Read the model definition and answer for the solid it produces. Units are mm, in the model's axes. Face numbers are marked on the shaded views. A direction names the side the tool comes from. Give positions to 0.01 mm unless a question says otherwise; leave off trailing zeros. Loops run counter-clockwise (first coordinate to the right, second up) from the corner with the lowest first, then second, coordinate; pieces in that order, holes last. Notation, with made-up numbers: (13, -18.5) - (35, -18.5) arc R27 ccw to (35, 1.5) - close; hole circle Ø1 at (-17, 5.25). An arc over 180 degrees is marked (long way). Put each result on its own line as item: value. Start each with the question number.
1. Given pin 1 Ø3 at (x, y) = (7.5, -32) entering from -Z; pin 2 Ø2.5 at (y, z) = (29.5, 2.5) entering from -X; pin 3 Ø4 at (x, z) = (-21, 4.5) entering from +Y; pin 4 Ø10 at (x, y) = (-1.5, 14) entering from -Z, each flat-ended and moving along its own axis, determine where each tip first touches the part or whether it passes through.
2. A cutting plane is placed at C-C, the plane y = 16.5. Determine the outline of the cut face in (x, z).
3. Consider L1, parallel to X at y = -32, z = 3; L2, parallel to Y at x = -16, z = 3.75; L3, parallel to Y at x = 15, z = 4.5. Determine where each line is inside the solid, lowest interval first. Write a range as from..to.
4. A cutting plane is placed at B-B, the plane x = 15. Determine the outline of the cut face in (y, z), plus the area to 3 significant figures.
5. For the marked faces 5 and 6, determine the directions among +Z, -Z, +X, -X, +Y, -Y from which every point of the face is accessible in a straight line to the end or side of a thin tool.
6. A cutting plane is placed at A-A, the plane y = 1. Determine the outline of the cut face in (x, z), plus the area to 3 significant figures.
7. A cutting plane is placed at D-D, the plane z = 6.75. Count the separate pieces of the cut face and the enclosed holes in it, plus the area to 3 significant figures.
8. For a pull along Y with two mould halves and no side action, classify the marked faces 1, 2, 3 and 4 as released by +Y, released by -Y, zero draft, split by the parting line, or undercut.
Autodesk Inventor part; units mm, degrees
ref_plane "YZ Plane" through (0, 0, 0) normal (1, 0, 0) x (0, 1, 0)
ref_plane "XZ Plane" through (0, 0, 0) normal (0, 1, 0) x (-1, 0, 0)
ref_plane "XY Plane" through (0, 0, 0) normal (0, 0, 1) x (1, 0, 0)
sketch "Sketch1" plane through (0, 0, 0) normal (0, 0, 1) x (1, 0, 0)
  line L0 (-32.5, 20) -> (32.5, 20)
  line L1 (32.5, 20) -> (32.5, -20)
  line L2 (32.5, -20) -> (-32.5, -20)
  line L3 (-32.5, -20) -> (-32.5, 20)
  point P0 (0, 0)
  point P1 (0, 20)
  point P2 (-32.5, 0)
  dimension "d0" = 65
  dimension "d1" = 40
extrude "Extrusion1" add sketch "Sketch1" along normal blind 8
sketch "Sketch5" plane through (0, 0, 0) normal (0, 0, -1) x (-1, 0, 0)
  line L0 (-32.5, 40) -> (0.5, 40)
  line L1 (0.5, 40) -> (0.5, -40)
  line L2 (0.5, -40) -> (-32.5, -40)
  line L3 (-32.5, -40) -> (-32.5, 40)
  line L4 (-32.5, -20) -> (-32.5, 20)
  line L5 (-32.5, 20) -> (32.5, 20)
  line L6 (32.5, -20) -> (-32.5, -20)
  point P0 (0, 0)
  dimension "d22" = 20
  dimension "d23" = 20
  dimension "d24" = 33
extrude "Extrusion5" add sketch "Sketch5" against normal up to surface (8 mm away)
sketch "Sketch6" plane through (0, 0, 0) normal (0, 0, -1) x (-1, 0, 0)
  line L0 (0.5, 40) -> (-32.5, 40)
  line L1 (-32.5, 40) -> (-32.5, -40)
  line L2 (-15, 16.5) -> (16, 16.5) construction
  line L3 (16, 16.5) -> (16, -14.5) construction
  line L4 (16, -14.5) -> (-15, -14.5) construction
  line L5 (-15, -14.5) -> (-15, 16.5) construction
  line L6 (-15, 16.5) -> (16, -14.5) construction
  line L7 (16, 16.5) -> (-15, -14.5) construction
  circle A0 centre (-15, 16.5) radius 1.75
  circle A1 centre (16, 16.5) radius 1.75
  circle A2 centre (16, -14.5) radius 1.75
  circle A3 centre (-15, -14.5) radius 1.75
  circle A4 centre (0.5, 1) radius 8.5
  dimension "d29" = 31
  dimension "d30" = 33
  dimension "d31" = 39
  dimension "d32" = 3.5
  dimension "d33" = 17
extrude "Extrusion6" cut sketch "Sketch6" against normal blind 10
sketch "Sketch7" plane through (0, 0, 0) normal (0, 0, -1) x (-1, 0, 0)
  line L0 (-32.5, 40) -> (-32.5, -40)
  line L1 (0.5, 40) -> (-32.5, 40)
  line L2 (0.5, 20) -> (0.5, 40)
  line L3 (-32.5, -40) -> (0.5, -40)
  point P0 (0, 0)
  point P1 (-24.5, 32)
  point P2 (-7.5, 32)
  point P3 (-24.5, -32)
  point P4 (-7.5, -32)
  dimension "d36" = 8
  dimension "d37" = 8
  dimension "d38" = 8
  dimension "d39" = 17
  dimension "d40" = 8
  dimension "d41" = 64
hole "Hole1" at (24.5, 32, 0) direction (0, 0, 1) diameter 5 end through all
pattern_linear "Rectangular Pattern1" count 2 spacing 64 along (0, -1, 0) count 2 spacing 17 along (-1, 0, 0) of "Hole1"
fillet "Fillet1" radius 1.5 2 edges at (-0.5, -20, 4) (-0.5, 20, 4)
equation "\"d23\" = d22"
properties part number "0005-10-023 Suport motor x" material "Wood (Maple)"
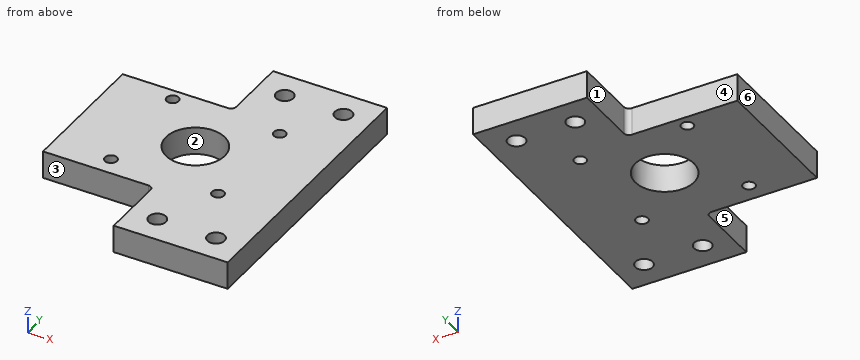
Return value:
1. pin 1: passes through
1. pin 2: stops at x = -0.5
1. pin 3: stops at y = 20
1. pin 4: stops at z = 0
2. outline: (-32.5, 0) - (-17.75, 0) - (-17.75, 8) - (-32.5, 8) - close; (-14.25, 0) - (13.25, 0) - (13.25, 8) - (-14.25, 8) - close; (16.75, 0) - (32.5, 0) - (32.5, 8) - (16.75, 8) - close
3. L1: x = -0.5..5, 10..22, 27..32.5
3. L2: y = -20..-16.25, -12.75..14.75, 18.25..20
3. L3: y = -40..-16.25, -12.75..14.75, 18.25..40
4. outline: (-40, 0) - (-16.25, 0) - (-16.25, 8) - (-40, 8) - close; (-12.75, 0) - (14.75, 0) - (14.75, 8) - (-12.75, 8) - close; (18.25, 0) - (40, 0) - (40, 8) - (18.25, 8) - close
4. area: 584 mm2
5. face 5: +Z, -Z, -X, -Y
5. face 6: +Z, -Z, -X, +Y, -Y
6. outline: (-32.5, 0) - (-9, 0) - (-9, 8) - (-32.5, 8) - close; (8, 0) - (32.5, 0) - (32.5, 8) - (8, 8) - close
6. area: 384 mm2
7. separate pieces: 1
7. enclosed holes: 9
7. area: 3,580 mm2
8. face 1: zero draft
8. face 2: undercut
8. face 3: released by -Y
8. face 4: released by +Y
